Model file for the job. Use its own axes, mm. A direction names the side the tool comes from. Coordinates: 2 decimals unless noted, no trailing zeros. Order: outer loops, then holes, each group sorted by start corner. A loop starts at its lowest first (then second) coordinate and runs counter-clockwise, first axis right, second up. Notation, with made-up numbers: (57, 29.5) -> (96, 29.5) arc R27 cw to (96, 54.5) -> close; hole circle Ø6 at (78, 25.5). An arc over 180 degrees is marked (long way). Write item = value, one per line. Start each with the question number.
Q1. 3-axis set-ups, long thin cutter, end or side, ignore diameter. For faces 1 (the face through (-5, 0, 4)), 2 (the face through (0, 12.75, 15)), 3 (the face through (0, 10, 24.8)): which of +Z, -Z, +X, -X, +Y, -Y reach the whole face in a straight line?
Q2. Cut at D-D, the plane x = -21. List the corners of the cut face in (y, z).
Q3. Cut at C-C, the plane z = 16.75. List the corners of the cut face in (x, y), plus the area to 3 significant figures.
Q4. Cut at A-A, the plane y = 19. List the corners of the cut face in (x, z), plus the area to 3 significant figures.
Q5. Mould opens along Z. For faces 4 (the face through (0, 12.75, 26)), 5 (the face through (0, 0, 26.8)), 6 (the face through (0, 10, 21.8)) say: +Z half, -Z half, draft (parallel to the pull), parting line (faces both ways), or undercut.
Q6. Flat gauge pins, fed straight in: pin 1 (1.5 mm diameter, centred on y = -13.5, z = 14, fed in from +X); pin 2 (14.5 mm diameter, centred on y = 20, z = 15.5, fed in from +X); pin 3 (1.2 mm diameter, centred on x = 5.5, y = 22, fed in from +Z). Where does each tip first touch, or does it go through?
Q7. Wall check: line 1 (Y direction, x = 0.5, z = 11.5); line 2 (X direction, y = -16, z = 8.25); line 3 (X direction, y = 23.5, z = 20). Give the ranges that are in metal, low to high. Write a range as from..to.
Q8. Cut at B-B, the plane y = -10. List the corners of the cut face in (x, z), plus the area to 3 significant figures.
from build123d import *

# Parameters (mm, degrees)
F0_W      = 20.5
F0_H      = 51.5
F0_W_2    = 19.25
F1_DEPTH  = 26.8
F2_W      = 13
F2_H      = 13
F3_DEPTH  = 26.8
F4_W      = 1.5
F4_H      = 13
F5_DEPTH  = 4.05
F7_DEPTH  = 51.501
F8_W      = 10
F8_H      = 8.67
F9_DEPTH  = 38.501
F10_W     = 13
F10_H     = 3
F11_DEPTH = 5


with BuildPart() as f1:
    # F0 (on Top) → F1 (new body)
    with BuildSketch(Plane.XY):
        Rectangle(F0_W, F0_H)
        with Locations((-19.875, 0)):
            Rectangle(F0_W_2, F0_H)
        with Locations((19.875, 0)):
            Rectangle(F0_W_2, F0_H)
    extrude(amount=F1_DEPTH)

    # F2 (on Top) → F3 (cut)
    with BuildSketch(Plane.XY):
        with Locations((0, 19.25)):
            Rectangle(F2_W, F2_H)
    extrude(amount=F3_DEPTH, mode=Mode.SUBTRACT)

    # F4 (on face) → F5 (join)
    with BuildSketch(Plane.XY):
        with Locations((-5.75, 19.25)):
            Rectangle(F4_W, F4_H)
        with Locations((5.75, 19.25)):
            Rectangle(F4_W, F4_H)
    extrude(amount=F5_DEPTH)

    # F6 (on face) → F7 (cut, through all)
    with BuildSketch(Plane(origin=(0, 25.75, 0), x_dir=(-1, 0, 0), z_dir=(0, 1, 0))):
        Polygon((10.244871, 26.8), (29.5, 0), (29.5, 26.8), align=None)
        Polygon((-29.5, 0), (-10.244871, 26.8), (-29.5, 26.8), align=None)
    extrude(amount=-F7_DEPTH, mode=Mode.SUBTRACT)

    # F8 (on face) → F9 (cut, through all)
    with BuildSketch(Plane(origin=(0, 12.75, 0), x_dir=(-1, 0, 0), z_dir=(0, 1, 0))):
        with Locations((0, 4.335)):
            Rectangle(F8_W, F8_H)
    extrude(amount=-F9_DEPTH, mode=Mode.SUBTRACT)

    # F10 (on face) → F11 (cut)
    with BuildSketch(Plane(origin=(0, 12.75, 0), x_dir=(-1, 0, 0), z_dir=(0, 1, 0))):
        with Locations((0, 23.3)):
            Rectangle(F10_W, F10_H)
    extrude(amount=-F11_DEPTH, mode=Mode.SUBTRACT)


solid = f1.part
Here are the results:
q1.face_1 = -Z, +Y, -Y
q1.face_2 = +Z, +Y
q1.face_3 = +Y
q2.outline = (-25.75, 0) -> (25.75, 0) -> (25.75, 11.83) -> (-25.75, 11.83) -> close
q3.outline = (-17.47, -25.75) -> (17.47, -25.75) -> (17.47, 25.75) -> (6.5, 25.75) -> (6.5, 12.75) -> (-6.5, 12.75) -> (-6.5, 25.75) -> (-17.47, 25.75) -> close
q3.area = 1,630 mm²
q4.outline = (-29.5, 0) -> (-5, 0) -> (-5, 4.05) -> (-6.5, 4.05) -> (-6.5, 26.8) -> (-10.24, 26.8) -> close; (5, 0) -> (29.5, 0) -> (10.24, 26.8) -> (6.5, 26.8) -> (6.5, 4.05) -> (5, 4.05) -> close
q4.area = 729 mm²
q5.face_4 = draft
q5.face_5 = +Z half
q5.face_6 = undercut
q6.pin_1 = 19.98
q6.pin_2 = 23.57
q6.pin_3 = 4.05
q7.line_1 = -25.75..12.75
q7.line_2 = -23.57..-5, 5..23.57
q7.line_3 = -15.13..-6.5, 6.5..15.13
q8.outline = (-29.5, 0) -> (-5, 0) -> (-5, 8.67) -> (5, 8.67) -> (5, 0) -> (29.5, 0) -> (10.24, 26.8) -> (-10.24, 26.8) -> close
q8.area = 978 mm²
